```python
from build123d import *

# Parameters (mm, degrees)
BOSS_EXTRUDE2_DEPTH = 25.4
SKETCH3_W           = 2.54
SKETCH3_H           = 20.32
CUT_EXTRUDE1_DEPTH  = 3.81
SKETCH4_R           = 1.190625
CUT_EXTRUDE2_DEPTH  = 30.934976745


with BuildPart() as part:
    # Sketch2 → Boss-Extrude2 (new body)
    with BuildSketch(Plane.XY):
        Polygon((-5, 4.637749078), (-7.54, 4.637749078), (-7.54, -4.851436151), (7.54, -4.851436151), (7.54, 4.637749078), (5, 4.637749078), (2.5, 2.54), (2.5, 0), (-2.5, 0), (-2.5, 2.54), align=None)
    extrude(amount=BOSS_EXTRUDE2_DEPTH)

    # Sketch3 → Cut-Extrude1 (cut)
    with BuildSketch(Plane(origin=(0, 0, 0), x_dir=(1, 0, 0), z_dir=(0, 1, 0))):
        with Locations((0, -15.24)):
            Rectangle(SKETCH3_W, SKETCH3_H)
    extrude(amount=-CUT_EXTRUDE1_DEPTH, mode=Mode.SUBTRACT)

    # Sketch4 → Cut-Extrude2 (cut, through all)
    with BuildSketch(Plane(origin=(7.54, 0, 0), x_dir=(0, 0, -1), z_dir=(1, 0, 0))):
        with Locations(Location((-17.78, 2.097749078, 0), (0, 0, 90))):
            Circle(SKETCH4_R)
    extrude(amount=-CUT_EXTRUDE2_DEPTH, mode=Mode.SUBTRACT)


solid = part.part
```
Geometry: final body of the model. Coordinates: model frame, mm. A direction names the side the tool comes from. Coordinates: 2 decimals unless noted, no trailing zeros. Order: outer loops, then holes, each group sorted by start corner. A loop starts at its lowest first (then second) coordinate and runs counter-clockwise, first axis right, second up. Notation, with made-up numbers: (66.25, -35.75) - (74.25, -35.75) arc R25 ccw to (74.25, -4.75) - close; hole circle Ø5 at (53.5, 34.5). An arc over 180 degrees is marked (long way). Return JSON: item names as keys, results as strings. Group by question number.
1. Cut plane C-C (y = -2). Output: boundary loops of the cut face in (x, z), plus the area to 3 significant figures.
2. Cut plane D-D (z = 17.78). Output: boundary loops of the cut face in (x, y).
3. Set-up query: faces 1 (the face through (3.767, 3.604, 12.522)), 2 (the face through (-1.27, -2, 15)), 3 (the face through (7.54, 0, 13)). Return all of +Z, -Z, +X, -X, +Y, -Y with unobstructed straight access to the full face (end or side cutting, diameter ignored); none if empty.
4. Pull-direction query (Z, two-part tool) for faces 4 (the face through (-7.54, 0, 13)), 5 (the face through (-4.98, 0.91, 17.83)), 6 (the face through (0, -2, 5.08)); classes: pulls with the +Z half, pulls with the -Z half, needs draft (parallel to the pull), parting line crosses it, or undercut.
5. Pin query (flat end, axial travel): pin 1 (3 mm diameter, centred on y = 2.1, z = 17.78, fed in from +X); pin 2 (2.5 mm diameter, centred on x = 0.5, z = 18, fed in from +Y); pin 3 (0.8 mm diameter, centred on x = 0.5, z = 10.5, fed in from +Y); pin 4 (0.8 mm diameter, centred on x = 0, y = -1.5, fed in from +Z). Return the tip coordinate at first contact, or that it passes through.
6. Material intervals for line 1 along X through (y, z) = (-2.5, 6); line 2 along Z through (x, y) = (5, 2); line 3 along Y through (x, z) = (5.05, 17.78), sorted ascending. Write a range as [from, to].
7. Cut plane B-B (z = 15). Output: boundary loops of the cut face in (x, y), plus the area to 3 significant figures.
8. Cut plane A-A (x = 5.5). Output: boundary loops of the cut face in (y, z), plus the area to 3 significant figures.
Resolved:
{
 "1": {"outline": "(-7.54, 0) - (7.54, 0) - (7.54, 25.4) - (1.27, 25.4) - (1.27, 5.08) - (-1.27, 5.08) - (-1.27, 25.4) - (-7.54, 25.4) - close", "area": "331 mm²"},
 "2": {"outline": "(-7.54, -4.85) - (7.54, -4.85) - (7.54, 0.91) - (2.5, 0.91) - (2.5, 0) - (1.27, 0) - (1.27, -3.81) - (-1.27, -3.81) - (-1.27, 0) - (-2.5, 0) - (-2.5, 0.91) - (-7.54, 0.91) - close; (-7.54, 3.29) - (-3.39, 3.29) - (-5, 4.64) - (-7.54, 4.64) - close; (3.39, 3.29) - (7.54, 3.29) - (7.54, 4.64) - (5, 4.64) - close"},
 "3": {"face 1": "+Z, -Z, +Y", "face 2": "+Z, +Y", "face 3": "+Z, -Z, +X, +Y, -Y"},
 "4": {"face 4": "needs draft", "face 5": "undercut", "face 6": "pulls with the +Z half"},
 "5": {"pin 1": "stops at x = 7.54", "pin 2": "stops at y = 0", "pin 3": "stops at y = -3.81", "pin 4": "stops at z = 5.08"},
 "6": {"line 1": "x = [-7.54, -1.27], [1.27, 7.54]", "line 2": "z = [0, 16.59], [18.97, 25.4]", "line 3": "y = [-4.85, 0.91], [3.29, 4.64]"},
 "7": {"outline": "(-7.54, -4.85) - (7.54, -4.85) - (7.54, 4.64) - (5, 4.64) - (2.5, 2.54) - (2.5, 0) - (1.27, 0) - (1.27, -3.81) - (-1.27, -3.81) - (-1.27, 0) - (-2.5, 0) - (-2.5, 2.54) - (-5, 4.64) - (-7.54, 4.64) - close", "area": "105 mm²"},
 "8": {"outline": "(-4.85, 0) - (4.64, 0) - (4.64, 25.4) - (-4.85, 25.4) - close; hole circle Ø2.38 at (2.1, 17.78)", "area": "237 mm²"}
}
